Could you check a few things on this model? Use its own coordinates, in mm. Face numbers are marked on the shaded views. A direction names the side the tool comes from. Coordinates: 2 decimals unless noted, no trailing zeros. Loops run counter-clockwise (first coordinate to the right, second up) from the corner with the lowest first, then second, coordinate; pieces in that order, holes last. Notation, with made-up numbers: (3.25, 15) - (43.25, 15) arc R14 ccw to (43.25, 40) - close; hole circle Ø6 at (5, -33). An arc over 180 degrees is marked (long way). Put each result on its own line as item: value. Start each with the question number.
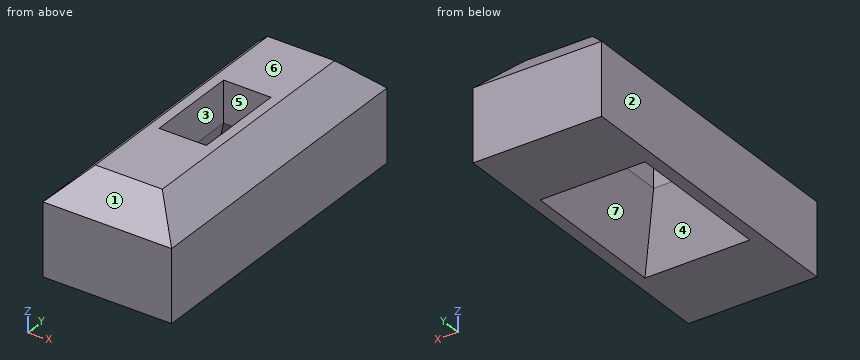
```python
from build123d import *
from OCP.BRepFilletAPI import BRepFilletAPI_MakeChamfer

# Parameters (mm, degrees)
ESBO_O1_W                = 12.5
ESBO_O1_H                = 30
RESSALTO_EXTRUS_O1_DEPTH = 10
ESBO_O2_W                = 4.6
ESBO_O2_H                = 9
CORTE_EXTRUS_O1_DEPTH    = 20.080421903
CHANFRO1_SIZE            = 3
CHANFRO2_SIZE            = 6
CHANFRO2_SIZE2           = 2.797845949


with BuildPart() as part:
    # Esboço1 → Ressalto-extrusão1 (new body)
    with BuildSketch(Plane.XY):
        Rectangle(ESBO_O1_W, ESBO_O1_H)
    extrude(amount=RESSALTO_EXTRUS_O1_DEPTH)

    # Esboço2 → Corte-extrusão1 (cut, through all)
    with BuildSketch(Plane.XY.offset(10)):
        Rectangle(ESBO_O2_W, ESBO_O2_H)
    extrude(amount=-CORTE_EXTRUS_O1_DEPTH, mode=Mode.SUBTRACT)

    # Chanfro1
    chanfro1_edges = [part.edges().sort_by_distance(p)[0] for p in [
        (-6.25, 0, 10),
        (0, -15, 10),
        (6.25, 0, 10),
        (0, 15, 10),
    ]]
    chamfer(chanfro1_edges, length=CHANFRO1_SIZE)

    # Chanfro2: one chamfer whose edges measure the first distance from different faces: ONE call of the kernel's chamfer builder (chamfer() names one face for all edges)
    chanfro2_edges_1 = [part.edges().sort_by_distance(p)[0] for p in [
        (2.3, 0, 0),
    ]]
    chanfro2_side_1 = [part.faces().sort_by_distance(p)[0] for p in [
        (2.3, 0, 5),
    ]]
    chanfro2_edges_2 = [part.edges().sort_by_distance(p)[0] for p in [
        (0, -4.5, 0),
    ]]
    chanfro2_side_2 = [part.faces().sort_by_distance(p)[0] for p in [
        (0, -4.5, 5),
    ]]
    chanfro2_edges_3 = [part.edges().sort_by_distance(p)[0] for p in [
        (-2.3, 0, 0),
    ]]
    chanfro2_side_3 = [part.faces().sort_by_distance(p)[0] for p in [
        (-2.3, 0, 5),
    ]]
    chanfro2_edges_4 = [part.edges().sort_by_distance(p)[0] for p in [
        (0, 4.5, 0),
    ]]
    chanfro2_side_4 = [part.faces().sort_by_distance(p)[0] for p in [
        (0, 4.5, 5),
    ]]
    chanfro2 = BRepFilletAPI_MakeChamfer(part.part.solid().wrapped)
    for e in chanfro2_edges_1:
        chanfro2.Add(CHANFRO2_SIZE, CHANFRO2_SIZE2, e.wrapped, chanfro2_side_1[0].wrapped)  # the first distance lies on this face
    for e in chanfro2_edges_2:
        chanfro2.Add(CHANFRO2_SIZE, CHANFRO2_SIZE2, e.wrapped, chanfro2_side_2[0].wrapped)  # the first distance lies on this face
    for e in chanfro2_edges_3:
        chanfro2.Add(CHANFRO2_SIZE, CHANFRO2_SIZE2, e.wrapped, chanfro2_side_3[0].wrapped)  # the first distance lies on this face
    for e in chanfro2_edges_4:
        chanfro2.Add(CHANFRO2_SIZE, CHANFRO2_SIZE2, e.wrapped, chanfro2_side_4[0].wrapped)  # the first distance lies on this face
    add(Compound.cast(chanfro2.Shape()), mode=Mode.REPLACE)


solid = part.part
```
(1) I want a section at B-B on x = -1. List the corners of the cut face in (y, z) for me, and give its area (3 significant figures).
(2) Which directions (+Z, -Z, +X, -X, +Y, -Y) give clear straight access to the entire face, cutting with the end or side of a thin tool? Please do the marked faces 5, 6 and 7.
(3) I want a section at C-C on z = 8. List the corners of the cut face in (x, y) for me.
(4) I need wall thicknesses on L1, parallel to X at y = -4.5, z = 2.5; L2, parallel to X at y = -5.5, z = 1.25; L3, parallel to Y at x = 1.25, z = 5.5. Which ranges of each line are inside material? Lowest first, please. Write a range as [from, to].
(5) I want a section at A-A on y = -1.75. List the corners of the cut face in (x, z) for me, and give its area (3 significant figures).
(6) For pin 1 Ø2 at (y, z) = (1, 9) entering from +X; pin 2 Ø2 at (x, z) = (-0.5, 9) entering from +Y; pin 3 Ø4 at (x, y) = (-3, 1) entering from -Z, each with a flat end and sliding along its axis, tell me the tip position at first contact or that it passes through.
(7) If we mould it in two halves opening along Y, with no side actions, what happens to the marked faces 1, 2, 3 and 4? For each: pulls with the +Y half, pulls with the -Y half, needs draft (parallel to the pull), parting line crosses it, or undercut.
(8) I want a section at D-D on y = -9.75. List the corners of the cut face in (x, z) for me, and give its area (3 significant figures).
Answer sheet:
1. outline: (-15, 0) - (-7.3, 0) - (-4.5, 6) - (-4.5, 10) - (-12, 10) - (-15, 7) - close; (4.5, 6) - (7.3, 0) - (15, 0) - (15, 7) - (12, 10) - (4.5, 10) - close
1. area: 184 mm^2
2. face 5: +Z, -Z
2. face 6: +Z, +X, -X, +Y, -Y
2. face 7: -Z
3. outline: (-5.25, -14) - (5.25, -14) - (5.25, 14) - (-5.25, 14) - close; hole (-2.3, -4.5) - (2.3, -4.5) - (2.3, 4.5) - (-2.3, 4.5) - close
4. L1: x = [-6.25, -3.93], [3.93, 6.25]
4. L2: x = [-6.25, -4.51], [4.51, 6.25]
4. L3: y = [-15, -4.73], [4.73, 15]
5. outline: (-6.25, 0) - (-5.1, 0) - (-2.3, 6) - (-2.3, 10) - (-3.25, 10) - (-6.25, 7) - close; (2.3, 6) - (5.1, 0) - (6.25, 0) - (6.25, 7) - (3.25, 10) - (2.3, 10) - close
5. area: 53.2 mm^2
6. pin 1: stops at x = 5.25
6. pin 2: stops at y = 14
6. pin 3: stops at z = 0.21
7. face 1: pulls with the -Y half
7. face 2: needs draft
7. face 3: undercut
7. face 4: undercut
8. outline: (-6.25, 0) - (6.25, 0) - (6.25, 7) - (3.25, 10) - (-3.25, 10) - (-6.25, 7) - close
8. area: 116 mm^2
